For this review, use the dimensioned drawing (mm, ordinates from the lowest corner) and the shaded views. Give positions to 0.01 mm unless a question says otherwise; leave off trailing zeros. Loops run counter-clockwise (first coordinate to the right, second up) from the corner with the lowest first, then second, coordinate; pieces in that order, holes last. Notation, with made-up numbers: M 32,-36.5 L 60,-36.5 A17 ccw 60,-21.5 Z; hole C -2.75,31.25 d5. An arc over 180 degrees is marked long. Use CSV: the item, a comma, the result in double quotes. Start each with the question number.
1. To check wall thickness, follow line 1 (Y direction, x = 59, z = 4.5); line 2 (Y direction, x = 88, z = 3.25); line 3 (Z direction, x = 53.5, y = 47). State the ranges of each line that lie inside material, in increasing order. Write a range as [from, to].
2. Take a section at A-A, the plane x = 20. Write out the cut boundary in (y, z).
3. Take a section at B-B, the plane z = 2.5. Write out the cut boundary in (x, y).
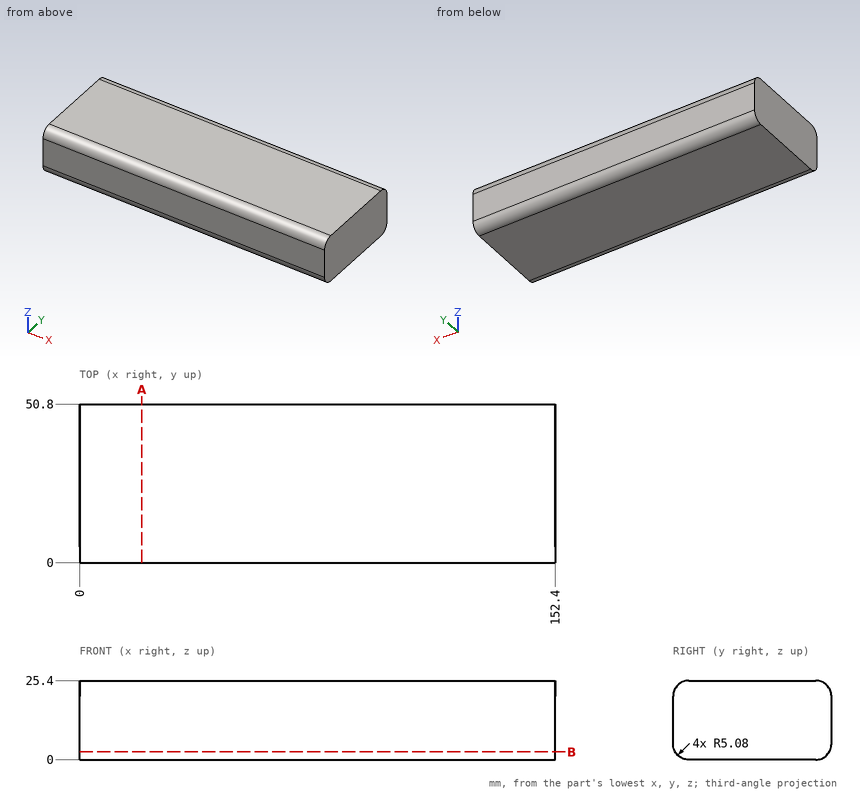
Result set:
1,line 1,"[0.03, 50.77]"
1,line 2,"[0.34, 50.46]"
1,line 3,"[0.16, 25.24]"
2,outline,"M 0,5.08 A5.08 ccw 5.08,0 L 45.72,0 A5.08 ccw 50.8,5.08 L 50.8,20.32 A5.08 ccw 45.72,25.4 L 5.08,25.4 A5.08 ccw 0,20.32 Z"
3,outline,"M 0,0.7 L 152.4,0.7 L 152.4,50.1 L 0,50.1 Z"
